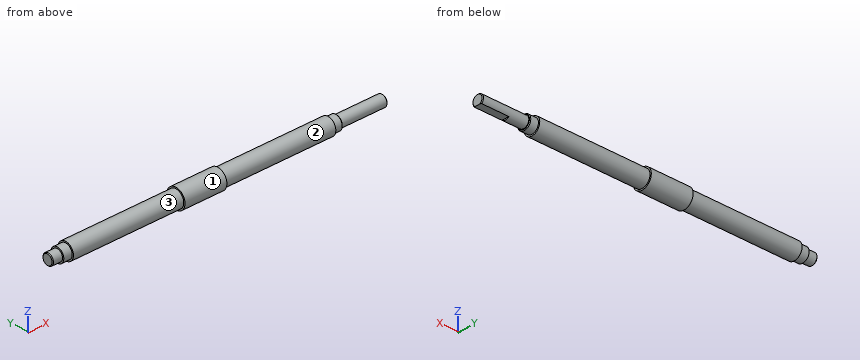
```python
from build123d import *

# Parameters (mm, degrees)
SKETCH_2_W          = 25.545670962
SKETCH_2_H          = 18.659121507
CUT_EXTRUDE_1_DEPTH = 10
CHAMFER_1_SIZE      = 0.5


with BuildPart() as part:
    # 草图1 → 旋转1 (revolve)
    with BuildSketch(Plane.XY):
        Polygon((-107, 0), (-107, 4), (-100, 4), (-100, 5), (-94, 5), (-94, 6), (-15, 6), (-15, 7), (15, 7), (15, 6), (94, 6), (94, 5), (100, 5), (100, 4), (133, 4), (133, 0), align=None)
    revolve(axis=Axis((-107, 0, 0), (1, 0, 0)))

    # 草图2 → 切除-拉伸1 (cut)
    with BuildSketch(Plane.XY.offset(-3)):
        with Locations((125.772835481, -0.110098382)):
            Rectangle(SKETCH_2_W, SKETCH_2_H)
    extrude(amount=-CUT_EXTRUDE_1_DEPTH, mode=Mode.SUBTRACT)

    # 倒角1
    chamfer_1_edges = [part.edges().sort_by_distance(p)[0] for p in [
        (100, -5, 0),
        (-107, -4, 0),
        (133, -1.645751311, 3.645751311),
    ]]
    chamfer(chamfer_1_edges, length=CHAMFER_1_SIZE)


solid = part.part
```
Geometry check sheet. Reference: the model listing, model coordinates, mm. Face numbers are marked on the shaded views. A direction names the side the tool comes from. Give positions to 0.01 mm unless a question says otherwise; leave off trailing zeros. Write each loop counter-clockwise with the first axis right and the second up, starting at its lowest first coordinate (ties: lowest second). Pieces come first, ordered by that corner, then holes.
1) Gauge pin test, flat ends, axial feed: pin 1 (8 mm diameter, centred on x = -64.5, z = 4, fed in from +Y); pin 2 (2 mm diameter, centred on x = 75, y = 5.5, fed in from +Z); pin 3 (1.5 mm diameter, centred on x = -37, y = 1, fed in from -Z). Record the tip position at first contact, or that the pin passes through.
2) Access from +Z, -Z, +X, -X, +Y, -Y to the whole of each face (thin tool, end or side, straight path). Record for the marked faces 1, 2 and 3.
3) Section check B-B, the plane x = -4.5. Record the boundary of the cut face in (y, z).
4) Material ranges on L1, parallel to Y at x = 107, z = 0.25; L2, parallel to Z at x = -76, y = 0; L3, parallel to X at y = 3.25, z = 3, recorded low to high.
5) Section check C-C, the plane x = -53. Record the boundary of the cut face in (y, z).
Computed:
1. pin 1: stops at y = 6
1. pin 2: stops at z = 3.97
1. pin 3: stops at z = -5.99
2. face 1: +X, -X
2. face 2: +X
2. face 3: -X
3. outline: circle Ø14 at (0, 0)
4. L1: y = -3.99 to 3.99
4. L2: z = -6 to 6
4. L3: x = -100 to 100
5. outline: circle Ø12 at (0, 0)
